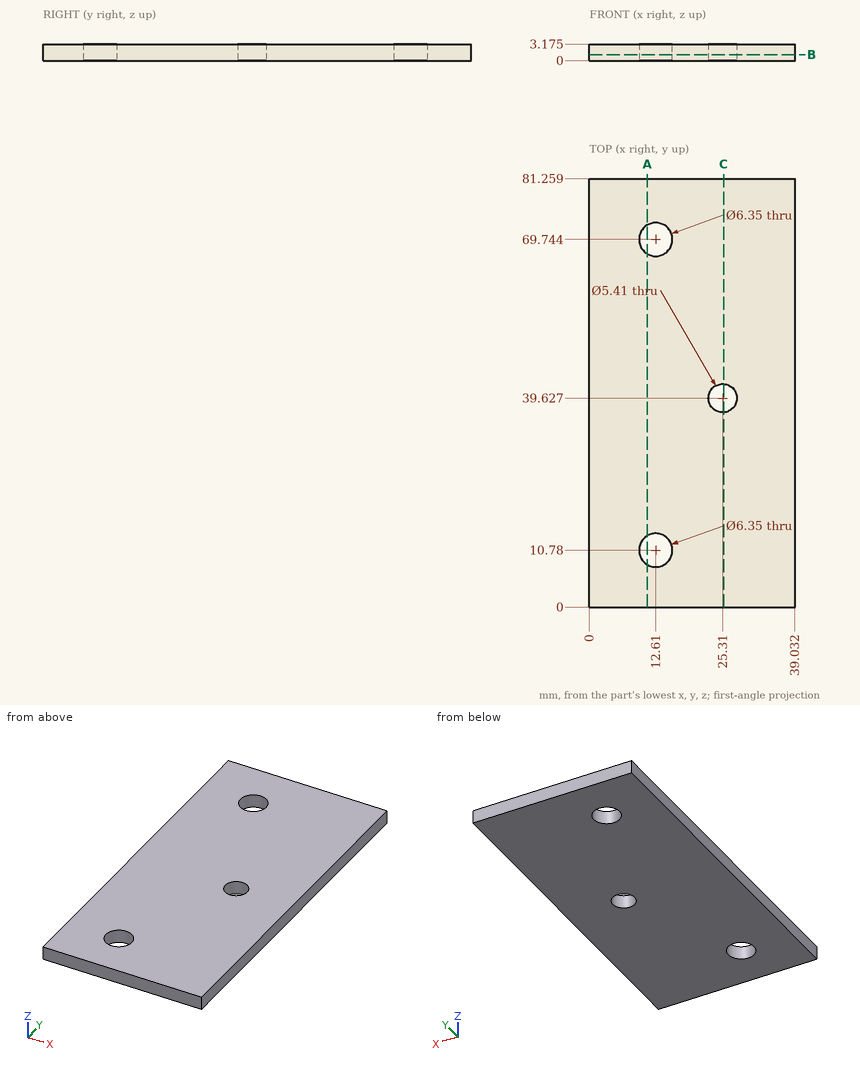
Geometry: see drawing. Coordinates: mm, zero at the bounding-box minimum. Round coordinates to 2 decimals unless told otherwise and drop trailing zeros. Order: outer loops, then holes, each group sorted by start corner. A loop starts at its lowest first (then second) coordinate and runs counter-clockwise, first axis right, second up. Notation, with made-up numbers: (59.25, -34) - (95.25, -34) arc R19 ccw to (95.25, -27) - close; hole circle Ø5 at (7.25, 16). An arc over 180 degrees is marked (long way). Use a Markdown table: item, result. Add a question column.
1. Section query C-C (x = 25.5). Return the cut outline in (y, z) (1 decimal), then the cut area to 3 significant figures.
2. Section query B-B (z = 1.15). Give the number of separate pieces and of enclosed holes in the cut face, then the cut area to 3 significant figures.
3. Section query A-A (x = 11). Return the cut outline in (y, z) (1 decimal), then the cut area to 3 significant figures.
4. Line query: probe 1 along X at (y, z) = (11, 2); probe 2 along Y at (x, z) = (12, 2.2) (1 decimal); probe 3 along X at (y, z) = (39.5, 1.2). Output: solid intervals per line, ascending.
Derived:
| question | item | result |
|---|---|---|
| 1 | outline | (0, 0) - (36.9, 0) - (36.9, 3.2) - (0, 3.2) - close; (42.3, 0) - (81.3, 0) - (81.3, 3.2) - (42.3, 3.2) - close |
| 1 | area | 241 mm2 |
| 2 | separate pieces | 1 |
| 2 | enclosed holes | 3 |
| 2 | area | 3,090 mm2 |
| 3 | outline | (0, 0) - (8, 0) - (8, 3.2) - (0, 3.2) - close; (13.5, 0) - (67, 0) - (67, 3.2) - (13.5, 3.2) - close; (72.5, 0) - (81.3, 0) - (81.3, 3.2) - (72.5, 3.2) - close |
| 3 | area | 223 mm2 |
| 4 | probe 1 | 0 to 9.44, 15.78 to 39.03 |
| 4 | probe 2 | 0 to 7.7, 13.9 to 66.6, 72.9 to 81.3 |
| 4 | probe 3 | 0 to 22.61, 28.01 to 39.03 |
